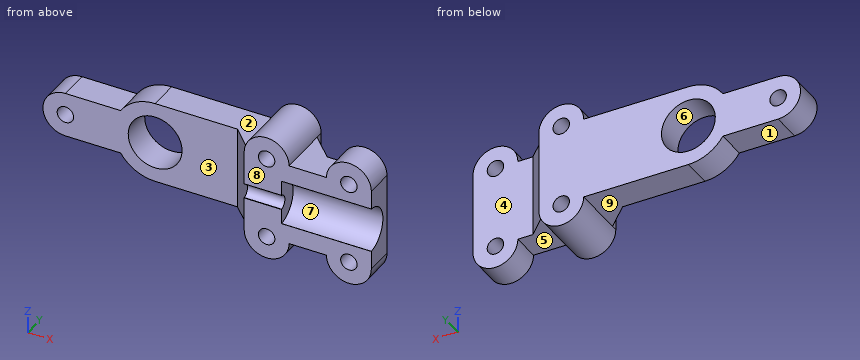
```python
from build123d import *

# Parameters (mm, degrees)
SKETCH_1_R              = 3
SKETCH_1_R_2            = 1.1
SKETCH_1_R_3            = 5.5
SKETCH_1_R_4            = 3.6
EXTRUDE_1_DEPTH         = 4
EXTRUDE_START           = 4
SKETCH_2_R              = 1.1
EXTRUDE_2_DEPTH         = 4
CHAMFER_1_SIZE          = 3
SKETCH_3_R              = 3
CUT_EXTRUDE_1_DEPTH     = 12
SKETCH_4_R              = 1
CUT_EXTRUDE_2_DEPTH     = 12
CHAMFER_2_SIZE          = 0.2
CUT_EXTRUDE_START       = -0.2
CUT_EXTRUDE_3_OUTLINE_R = 1.1
CUT_EXTRUDE_3_DEPTH     = 0.2


with BuildPart() as part:
    # 草图1 → 凸台-拉伸1 (new body)
    # profile 1 of 12: a face of its own
    with BuildSketch(Plane(origin=(0, 0, 0), x_dir=(1, 0, 0), z_dir=(0, 1, 0))):
        Circle(SKETCH_1_R)
        with Locations(Location((0, 0, 0), (0, 0, 270))):
            Circle(SKETCH_1_R_2, mode=Mode.SUBTRACT)
    # profile 2 of 12: a face of its own
    with BuildSketch(Plane(origin=(0, 0, 0), x_dir=(1, 0, 0), z_dir=(0, 1, 0))):
        with BuildLine():
            Line((7.390227771, 3), (0, 3))
            ThreePointArc((0, 3), (2.121320344, 2.121320344), (3, 0))
            ThreePointArc((3, 0), (2.121320344, -2.121320344), (0, -3))
            Line((0, -3), (7.390227771, -3))
            ThreePointArc((7.390227771, -3), (6.5, 0), (7.390227771, 3))
        make_face()
    # profile 3 of 12: a face of its own
    with BuildSketch(Plane(origin=(0, 0, 0), x_dir=(1, 0, 0), z_dir=(0, 1, 0))):
        with Locations((12, 0)):
            Circle(SKETCH_1_R_3)
        with Locations(Location((12, 0, 0), (0, 0, 270))):
            Circle(SKETCH_1_R_4, mode=Mode.SUBTRACT)
    # profile 4 of 12: a face of its own
    with BuildSketch(Plane(origin=(0, 0, 0), x_dir=(1, 0, 0), z_dir=(0, 1, 0))):
        with BuildLine():
            Line((26, 5.5), (12, 5.5))
            ThreePointArc((12, 5.5), (15.889087297, 3.889087297), (17.5, 0))
            ThreePointArc((17.5, 0), (15.889087297, -3.889087297), (12, -5.5))
            Line((12, -5.5), (26, -5.5))
            ThreePointArc((26, -5.5), (29, -2.5), (32, -5.5))
            Line((32, -5.5), (32, 5.5))
            ThreePointArc((32, 5.5), (29, 2.5), (26, 5.5))
        make_face()
    # profile 5 of 12: a face of its own
    with BuildSketch(Plane(origin=(0, 0, 0), x_dir=(1, 0, 0), z_dir=(0, 1, 0))):
        with BuildLine():
            ThreePointArc((32, 5.5), (29, 8.5), (26, 5.5))
            Line((26, 5.5), (27.9, 5.5))
            ThreePointArc((27.9, 5.5), (29, 6.6), (30.1, 5.5))
            Line((30.1, 5.5), (32, 5.5))
        make_face()
    # profile 6 of 12: a face of its own
    with BuildSketch(Plane(origin=(0, 0, 0), x_dir=(1, 0, 0), z_dir=(0, 1, 0))):
        with BuildLine():
            Line((27.9, 5.5), (26, 5.5))
            ThreePointArc((26, 5.5), (29, 2.5), (32, 5.5))
            Line((32, 5.5), (30.1, 5.5))
            ThreePointArc((30.1, 5.5), (29, 4.4), (27.9, 5.5))
        make_face()
    # profile 7 of 12: a face of its own
    with BuildSketch(Plane(origin=(0, 0, 0), x_dir=(1, 0, 0), z_dir=(0, 1, 0))):
        with BuildLine():
            ThreePointArc((32, 5.5), (29, 8.5), (26, 5.5))
            Line((26, 5.5), (27.9, 5.5))
            ThreePointArc((27.9, 5.5), (29, 6.6), (30.1, 5.5))
            Line((30.1, 5.5), (32, 5.5))
        make_face()
    # profile 8 of 12: a face of its own
    with BuildSketch(Plane(origin=(0, 0, 0), x_dir=(1, 0, 0), z_dir=(0, 1, 0))):
        with BuildLine():
            Line((27.9, 5.5), (26, 5.5))
            ThreePointArc((26, 5.5), (29, 2.5), (32, 5.5))
            Line((32, 5.5), (30.1, 5.5))
            ThreePointArc((30.1, 5.5), (29, 4.4), (27.9, 5.5))
        make_face()
    # profile 9 of 12: a face of its own
    with BuildSketch(Plane(origin=(0, 0, 0), x_dir=(1, 0, 0), z_dir=(0, 1, 0))):
        with BuildLine():
            ThreePointArc((32, -5.5), (29, -2.5), (26, -5.5))
            Line((26, -5.5), (27.9, -5.5))
            ThreePointArc((27.9, -5.5), (29, -4.4), (30.1, -5.5))
            Line((30.1, -5.5), (32, -5.5))
        make_face()
    # profile 10 of 12: a face of its own
    with BuildSketch(Plane(origin=(0, 0, 0), x_dir=(1, 0, 0), z_dir=(0, 1, 0))):
        with BuildLine():
            Line((27.9, -5.5), (26, -5.5))
            ThreePointArc((26, -5.5), (29, -8.5), (32, -5.5))
            Line((32, -5.5), (30.1, -5.5))
            ThreePointArc((30.1, -5.5), (29, -6.6), (27.9, -5.5))
        make_face()
    # profile 11 of 12: a face of its own
    with BuildSketch(Plane(origin=(0, 0, 0), x_dir=(1, 0, 0), z_dir=(0, 1, 0))):
        with BuildLine():
            ThreePointArc((32, -5.5), (29, -2.5), (26, -5.5))
            Line((26, -5.5), (27.9, -5.5))
            ThreePointArc((27.9, -5.5), (29, -4.4), (30.1, -5.5))
            Line((30.1, -5.5), (32, -5.5))
        make_face()
    # profile 12 of 12: a face of its own
    with BuildSketch(Plane(origin=(0, 0, 0), x_dir=(1, 0, 0), z_dir=(0, 1, 0))):
        with BuildLine():
            Line((27.9, -5.5), (26, -5.5))
            ThreePointArc((26, -5.5), (29, -8.5), (32, -5.5))
            Line((32, -5.5), (30.1, -5.5))
            ThreePointArc((30.1, -5.5), (29, -6.6), (27.9, -5.5))
        make_face()
    extrude(amount=EXTRUDE_1_DEPTH)

    # 草图2 → 凸台-拉伸2 (add)
    # profile 1 of 3: a face of its own
    with BuildSketch(Plane.XZ.offset(EXTRUDE_START)):
        with BuildLine():
            Line((26, 5.5), (26, -5.5))
            ThreePointArc((26, -5.5), (29, -8.5), (32, -5.5))
            Line((32, -5.5), (32, 5.5))
            ThreePointArc((32, 5.5), (29, 8.5), (26, 5.5))
        make_face()
        with Locations(Location((29, 5.5, 0), (0, 0, 270))):
            Circle(SKETCH_2_R, mode=Mode.SUBTRACT)
        with Locations(Location((29, -5.5, 0), (0, 0, 270))):
            Circle(SKETCH_2_R, mode=Mode.SUBTRACT)
    # profile 2 of 3: a face of its own
    with BuildSketch(Plane.XZ.offset(EXTRUDE_START)):
        with BuildLine():
            Line((37, 5.5), (32, 5.5))
            Line((32, 5.5), (32, 0))
            Line((32, 0), (43, 0))
            Line((43, 0), (43, 5.5))
            ThreePointArc((43, 5.5), (40, 8.5), (37, 5.5))
        make_face()
        with Locations(Location((40, 5.5, 0), (0, 0, 270))):
            Circle(SKETCH_2_R, mode=Mode.SUBTRACT)
    # profile 3 of 3: a face of its own
    with BuildSketch(Plane.XZ.offset(EXTRUDE_START)):
        with BuildLine():
            Line((32, 0), (32, -5.5))
            Line((32, -5.5), (37, -5.5))
            ThreePointArc((37, -5.5), (40, -8.5), (43, -5.5))
            Line((43, -5.5), (43, 0))
            Line((43, 0), (32, 0))
        make_face()
        with Locations(Location((40, -5.5, 0), (0, 0, 270))):
            Circle(SKETCH_2_R, mode=Mode.SUBTRACT)
    extrude(amount=-EXTRUDE_2_DEPTH)

    # 倒角1
    chamfer_1_edges = [part.edges().sort_by_distance(p)[0] for p in [
        (32, 0, 0),
        (26, 0, 0),
    ]]
    chamfer(chamfer_1_edges, length=CHAMFER_1_SIZE)

    # 草图3 → 切除-拉伸1 (cut)
    with BuildSketch(Plane(origin=(43, 0, 0), x_dir=(0, 0, -1), z_dir=(1, 0, 0))):
        with Locations((0, -4)):
            Circle(SKETCH_3_R)
    extrude(amount=-CUT_EXTRUDE_1_DEPTH, mode=Mode.SUBTRACT)

    # 草图4 → 切除-拉伸2 (cut)
    with BuildSketch(Plane(origin=(31, 0, 0), x_dir=(0, 0, -1), z_dir=(1, 0, 0))):
        with Locations((0, -4)):
            Circle(SKETCH_4_R)
    extrude(amount=-CUT_EXTRUDE_2_DEPTH, mode=Mode.SUBTRACT)

    # 倒角2
    # the kernel refuses this chamfer: 0.2 mm, written as the material it takes off along each edge
    with BuildSketch(Plane(origin=(31, -4, 3), x_dir=(0, 0, 1), z_dir=(1, 0, 0)), Plane(origin=(43.53300923, -4, -3), x_dir=(0, 0, -1), z_dir=(-1, 0, 0))) as chamfer_2_piece_1:
        with BuildLine():
            Line((CHAMFER_2_SIZE, 0), (-0.007161172, -0.207161172))
            ThreePointArc((-0.007161172, -0.207161172), (-0.001893441, -0.106569522), (0, 0))
            Line((0, 0), (CHAMFER_2_SIZE, 0))
        make_face()
    extrude(amount=12.53300923, mode=Mode.SUBTRACT)
    with BuildSketch(Plane(origin=(31.584058146, -4, -1), x_dir=(0, 0.9935204423355923, 0.11365355542739984), z_dir=(-1, 0, 0))) as chamfer_2_piece_2:
        with BuildLine():
            Line((0.227307111, 0), (-CHAMFER_2_SIZE * 0.113653555427, CHAMFER_2_SIZE * 0.993520442336))
            Line((-CHAMFER_2_SIZE * 0.113653555427, CHAMFER_2_SIZE * 0.993520442336), (0, 0))
            ThreePointArc((0, 0), (0.116813439, 0.006474565), (0.227307111, 0))
        make_face()
    extrude(amount=6.168116293, mode=Mode.SUBTRACT)
    with BuildSketch(Plane(origin=(25.415941854, -4, 1), x_dir=(0, 0, 1), z_dir=(1, 0, 0))) as chamfer_2_piece_3:
        with BuildLine():
            Line((CHAMFER_2_SIZE, 0), (-0.025834261, -0.225834261))
            ThreePointArc((-0.025834261, -0.225834261), (-0.00684365, -0.116792397), (0, 0))
            Line((0, 0), (CHAMFER_2_SIZE, 0))
        make_face()
    extrude(amount=6.168116293, mode=Mode.SUBTRACT)

    # 切除-拉伸3: read off the stored shape, not the designer's step
    # 切除-拉伸3 outline → 切除-拉伸3 (cut)
    with BuildSketch(Plane.XZ.offset(4).offset(CUT_EXTRUDE_START)):
        with BuildLine():
            Line((26, 5.5), (26, -5.5))
            ThreePointArc((26, -5.5), (29, -8.5), (32, -5.5))
            Line((32, -5.5), (37, -5.5))
            ThreePointArc((37, -5.5), (40, -8.5), (43, -5.5))
            Line((43, -5.5), (43, 5.5))
            ThreePointArc((43, 5.5), (40, 8.5), (37, 5.5))
            Line((37, 5.5), (32, 5.5))
            ThreePointArc((32, 5.5), (29, 8.5), (26, 5.5))
        make_face()
        with Locations((29, -5.5)):
            Circle(CUT_EXTRUDE_3_OUTLINE_R, mode=Mode.SUBTRACT)
        with Locations((40, -5.5)):
            Circle(CUT_EXTRUDE_3_OUTLINE_R, mode=Mode.SUBTRACT)
        with Locations((29, 5.5)):
            Circle(CUT_EXTRUDE_3_OUTLINE_R, mode=Mode.SUBTRACT)
        with Locations((40, 5.5)):
            Circle(CUT_EXTRUDE_3_OUTLINE_R, mode=Mode.SUBTRACT)
    extrude(amount=CUT_EXTRUDE_3_DEPTH, mode=Mode.SUBTRACT)


solid = part.part
```
Here's how the part is built. I have some questions about the finished solid (model axes, mm). Face numbers are marked on the shaded views. A direction names the side the tool comes from. Coordinates: 2 decimals unless noted, no trailing zeros. Order: outer loops, then holes, each group sorted by start corner. A loop starts at its lowest first (then second) coordinate and runs counter-clockwise, first axis right, second up.
1) Imagine slicing it at C-C on z = 7. List the corners of the cut face in (x, y) for me.
2) I need wall thicknesses on line 1 (Z direction, x = 29, y = 2.25); line 2 (X direction, y = 0.85, z = 0); line 3 (Z direction, x = 29.5, y = -2.25). Which ranges of each line are inside material? Lowest first, please.
3) Which directions (+Z, -Z, +X, -X, +Y, -Y) give clear straight access to the entire face, cutting with the end or side of a thin tool? Please do the marked faces 1, 2, 3, 4 and 5.
4) Will these pins go through, and if not, where does the flat tip stop? pin 1 (0.9 mm diameter, centred on y = -3.5, z = 2, fed in from -X); pin 2 (3.5 mm diameter, centred on x = 20, y = -0.5, fed in from +Z); pin 3 (5 mm diameter, centred on x = 7, z = -1.5, fed in from -Y); pin 4 (6 mm diameter, centred on x = 12, z = 0, fed in from +Y).
5) Imagine slicing it at D-D on z = -0.5. List the corners of the cut face in (x, y) for me.
6) Imagine slicing it at B-B on y = 0.5. List the corners of the cut face in (x, z) for me.
7) Imagine slicing it at A-A on x = 29. State how many separate pieces and enclosed holes the cut face has, and give its area (3 significant figures).
8) We'd pull the mould along Z, two halves only. Please class the marked faces 6, 7, 8 and 9: +Z half, -Z half, draft (parallel to the pull), parting line (faces both ways), or undercut.
Response values:
1. outline: (26.4, -3.8) - (31.6, -3.8) - (31.6, 4) - (26.4, 4) - close; (37.4, -3.8) - (42.6, -3.8) - (42.6, 0) - (37.4, 0) - close
2. line 1: z = -8.5 to -6.6, -4.4 to 4.4, 6.6 to 8.5
2. line 2: x = -3 to -1.1, 1.1 to 8.4, 15.6 to 34.15
2. line 3: z = -8.46 to -6.48, -4.52 to 4.52, 6.48 to 8.46
3. face 1: -Z, -X, +Y, -Y
3. face 2: +Z, -X, +Y, -Y
3. face 3: +Z, -Z, -X, -Y
3. face 4: +Z, -Z, +X, +Y
3. face 5: -Z, +Y, -Y
4. pin 1: stops at x = 26
4. pin 2: stops at z = 5.5
4. pin 3: stops at y = 0
4. pin 4: passes through
5. outline: (-2.96, 0) - (-0.98, 0) - (-0.98, 4) - (-2.96, 4) - close; (0.98, 0) - (8.43, 0) - (8.43, 4) - (0.98, 4) - close; (15.57, 0) - (23, 0) - (26, -3) - (26, -3.13) - (31, -3.13) - (31, -1.04) - (43, -1.04) - (43, 0) - (35, 0) - (32, 3) - (32, 4) - (15.57, 4) - close
6. outline: (0, -3) - (7.39, -3) arc R5.5 ccw to (12, -5.5) - (26, -5.5) arc R3 ccw to (32, -5.5) - (34.5, -5.5) - (34.5, 5.5) - (32, 5.5) arc R3 ccw to (26, 5.5) - (12, 5.5) arc R5.5 ccw to (7.39, 3) - (0, 3) arc R3 ccw to start; hole circle Ø2.2 at (0, 0); hole circle Ø7.2 at (12, 0); hole circle Ø2.2 at (29, -5.5); hole circle Ø2.2 at (29, 5.5)
7. separate pieces: 3
7. enclosed holes: 0
7. area: 97.1 mm2
8. face 6: undercut
8. face 7: undercut
8. face 8: draft
8. face 9: -Z half
